Design review of the part built by this model. Coordinates are the model's own, in mm. Face numbers are marked on the shaded views. A direction names the side the tool comes from. Coordinates: 2 decimals unless noted, no trailing zeros. Order: outer loops, then holes, each group sorted by start corner. A loop starts at its lowest first (then second) coordinate and runs counter-clockwise, first axis right, second up. Notation, with made-up numbers: (23.25, 4.25) - (75.25, 4.25) arc R21 ccw to (75.25, 41.25) - close; hole circle Ø2 at (-8, 38.25). An arc over 180 degrees is marked (long way). Write item = value, one per line. Start each with the question number.
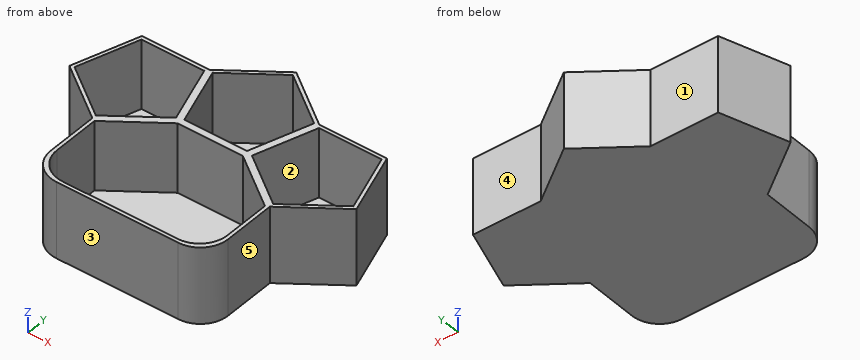
```python
from build123d import *

# Parameters (mm, degrees)
F1_DEPTH = 25.4
F3_DEPTH = 2.54
F4_R     = 10.16


with BuildPart() as f1:
    # F0 (on Top) → F1 (new body)
    with BuildSketch(Plane.XY):
        Polygon((44.789236, 6.508257), (20.030355, 6.508257), (12.37944, -17.038838), (32.409796, -31.591743), (52.440151, -17.038838), align=None)
        Polygon((20.953064, 5.238257), (43.866527, 5.238257), (50.947177, -16.553741), (32.409796, -30.021937), (13.872415, -16.553741), align=None, mode=Mode.SUBTRACT)
        Polygon((12.37944, -17.038838), (20.030355, 6.508257), (0, 21.061162), (-20.030355, 6.508257), (-12.37944, -17.038838), align=None)
        Polygon((-18.537381, 6.02316), (0, 19.491356), (18.537381, 6.02316), (11.456731, -15.768838), (-11.456731, -15.768838), align=None, mode=Mode.SUBTRACT)
        Polygon((32.409796, -31.591743), (12.37944, -17.038838), (-12.37944, -17.038838), (-32.409796, -31.591743), (-32.409796, -60.778446), (32.409796, -60.778446), align=None)
        Polygon((31.139796, -32.23884), (31.139796, -59.508446), (-31.139796, -59.508446), (-31.139796, -32.23884), (-11.966792, -18.308838), (11.966792, -18.308838), align=None, mode=Mode.SUBTRACT)
        Polygon((-32.409796, -31.591743), (-12.37944, -17.038838), (-20.030355, 6.508257), (-44.789236, 6.508257), (-52.440151, -17.038838), align=None)
        Polygon((-43.866527, 5.238257), (-20.953064, 5.238257), (-13.872415, -16.553741), (-32.409796, -30.021937), (-50.947177, -16.553741), align=None, mode=Mode.SUBTRACT)
    extrude(amount=F1_DEPTH)

    # F2 (on Top) → F3 (join)
    with BuildSketch(Plane.XY):
        Polygon((0, 21.061162), (-20.030355, 6.508257), (-44.789236, 6.508257), (-52.440151, -17.038838), (-32.409796, -31.591743), (-32.409796, -60.778446), (32.409796, -60.778446), (32.409796, -31.591743), (52.440151, -17.038838), (44.789236, 6.508257), (20.030355, 6.508257), align=None)
    extrude(amount=-F3_DEPTH)

    # F4
    f4_edges = [f1.edges().sort_by_distance(p)[0] for p in [
        (32.409796, -60.778446, 11.43),
        (-32.409796, -60.778446, 11.43),
        (-31.139796, -59.508446, 12.7),
        (31.139796, -59.508446, 12.7),
    ]]
    fillet(f4_edges, radius=F4_R)


solid = f1.part
```
Item 1: Add section D-D on x = 6. Give the boundary of the cut face in (y, z), plus the area to 3 significant figures.
Item 2: Add section A-A on x = -27. Give the boundary of the cut face in (y, z), plus the area to 3 significant figures.
Item 3: For the marked faces 1, 2, 3, 4 and 5, list the 3-axis set-ups (+Z, -Z, +X, -X, +Y, -Y) from which the entire face can be reached by the end or side of a thin tool; tool diameter is ignored.
Item 4: For P1, Ø4, axis at y = 0.5, z = 6.5, coming from the +X side; P2, Ø7.5, axis at x = -32.5, z = 4.5, coming from the +Y side; P3, Ø2, axis at y = -32.5, z = 8, coming from the -X side; P4, Ø11.5, axis at x = -0.5, z = 8.5, coming from the +Y side, all flat-tipped, find the tip position at first contact; note any pin that passes through.
Item 5: For line 1 (X direction, y = -38.5, z = 4.5); line 2 (X direction, y = -4.5, z = 10.5); line 3 (Y direction, x = -8.5, z = 24.25), list the stretches that pass through material, from the lowest coordinate up.
Item 6: Add section C-C on z = 21.5. State how many separate pieces and enclosed holes the cut face has, plus the area to 3 significant figures.
Item 7: Add section B-B on y = -10. Give the boundary of the cut face in (x, z), plus the area to 3 significant figures.
Worked out:
q1.outline = (-60.78, -2.54) - (16.7, -2.54) - (16.7, 25.4) - (15.13, 25.4) - (15.13, 0) - (-15.77, 0) - (-15.77, 25.4) - (-18.31, 25.4) - (-18.31, 0) - (-59.51, 0) - (-59.51, 25.4) - (-60.78, 25.4) - close
q1.area = 333 mm2
q2.outline = (-59.6, -2.54) - (6.51, -2.54) - (6.51, 25.4) - (5.24, 25.4) - (5.24, 0) - (-26.09, 0) - (-26.09, 25.4) - (-29.23, 25.4) - (-29.23, 0) - (-57.53, 0) - (-57.53, 25.4) - (-59.6, 25.4) - close
q2.area = 332 mm2
q3.face_1 = +Z, -Z, -X, +Y
q3.face_2 = +Z
q3.face_3 = +Z, -Z, +X, -X, -Y
q3.face_4 = +Z, -Z, +X, +Y
q3.face_5 = +Z, -Z, +X, -Y
q4.P1 = 47.39
q4.P2 = 6.51
q4.P3 = -32.54
q4.P4 = 21.06
q5.line_1 = -32.41 to -31.14, 31.14 to 32.41
q5.line_2 = -48.37 to -47.03, -17.79 to -15.12, 15.12 to 17.79, 47.03 to 48.37
q5.line_3 = -60.78 to -59.51, -18.31 to -15.77, 13.32 to 14.89
q6.separate_pieces = 1
q6.enclosed_holes = 4
q6.area = 699 mm2
q7.outline = (-50.15, -2.54) - (50.15, -2.54) - (50.15, 25.4) - (48.82, 25.4) - (48.82, 0) - (16, 0) - (16, 25.4) - (13.33, 25.4) - (13.33, 0) - (-13.33, 0) - (-13.33, 25.4) - (-16, 25.4) - (-16, 0) - (-48.82, 0) - (-48.82, 25.4) - (-50.15, 25.4) - close
q7.area = 458 mm2
